The drawing under review shows one solid part. Ordinate dimensions are in mm from its lowest x, y, z. A direction names the side the tool comes from. Coordinates: 2 decimals unless noted, no trailing zeros. Order: outer loops, then holes, each group sorted by start corner. A loop starts at its lowest first (then second) coordinate and runs counter-clockwise, first axis right, second up.
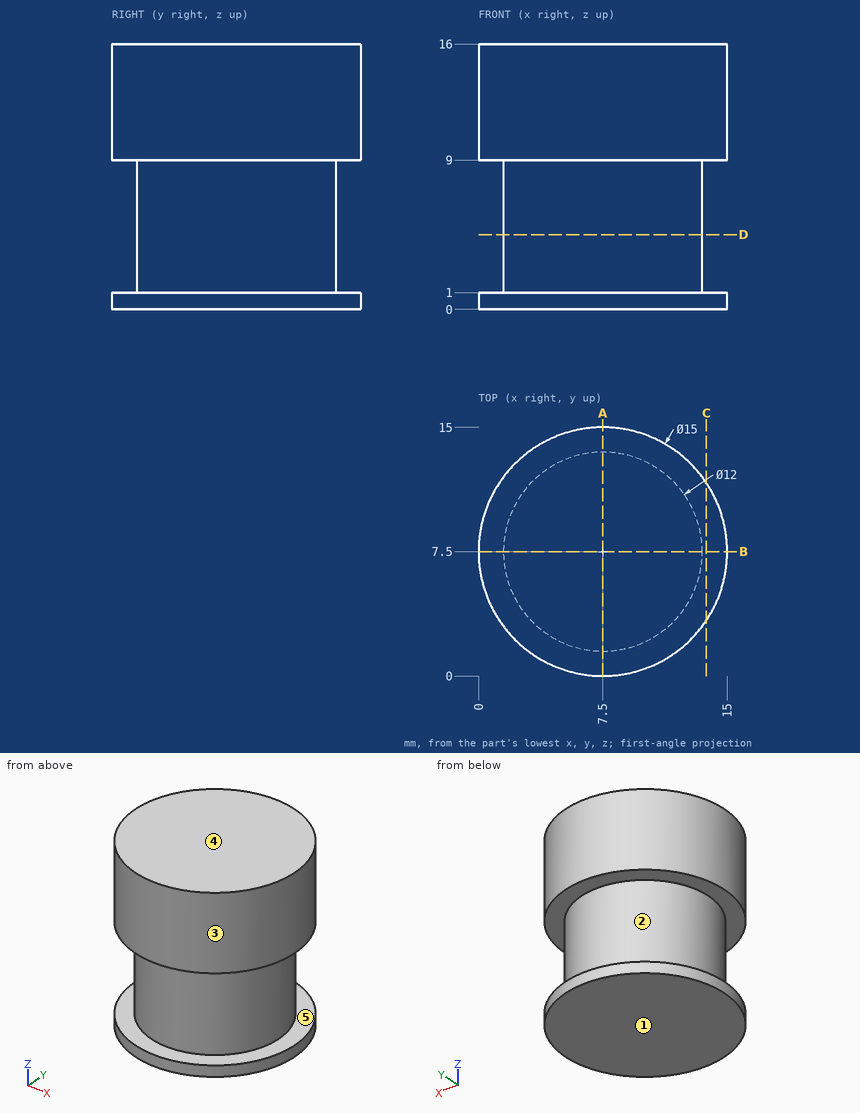
(1) We need section A-A, the plane x = 7.5. Write out the cut boundary in (y, z), and give its area (3 significant figures).
A:
outline: (0, 0) - (15, 0) - (15, 1) - (13.5, 1) - (13.5, 9) - (15, 9) - (15, 16) - (0, 16) - (0, 9) - (1.5, 9) - (1.5, 1) - (0, 1) - close
area: 216 mm2
(2) For pin 1 Ø8 at (x, y) = (5.5, 11.5) entering from -Z; pin 2 Ø1.5 at (x, z) = (11, 8) entering from +Y, all flat-tipped, find the tip position at first contact; note any pin that passes through.
A:
pin 1: stops at z = 0
pin 2: stops at y = 12.83
(3) We need section D-D, the plane z = 4.5. Write out the cut boundary in (x, y), and give its area (3 significant figures).
A:
outline: circle Ø12 at (7.5, 7.5)
area: 113 mm2
(4) Wall thickness on probe 1 along Z at (x, y) = (1.5, 9.5); probe 2 along X at (y, z) = (7.75, 7.25); probe 3 along Y at (x, z) = (7.5, 8.5): over which ranges is each line inside the solid? List them lowest first.
A:
probe 1: z = 0 to 1, 9 to 16
probe 2: x = 1.51 to 13.49
probe 3: y = 1.5 to 13.5
(5) Draft analysis for pull direction Z (two halves, no side actions). For the marked faces 1, 2 and 3, state which applies: released by +Z, released by -Z, zero draft, split by the parting line, or undercut.
A:
face 1: released by -Z
face 2: undercut
face 3: zero draft
(6) Machinability: for the marked faces 4 and 5, which of the approach directions +Z, -Z, +X, -X, +Y, -Y give a long, thin tool a straight path to every point of the face, cutting with its end or side? Answer none if there is none.
A:
face 4: +Z, +X, -X, +Y, -Y
face 5: none
(7) We need section C-C, the plane x = 13.75. Write out the cut boundary in (y, z).
A:
outline: (3.35, 0) - (11.65, 0) - (11.65, 1) - (3.35, 1) - close; (3.35, 9) - (11.65, 9) - (11.65, 16) - (3.35, 16) - close
